The model under review builds one solid part; all positions refer to its coordinate system, in mm. Coordinates: 2 decimals unless noted, no trailing zeros. Write each loop counter-clockwise with the first axis right and the second up, starting at its lowest first coordinate (ties: lowest second). Pieces come first, ordered by that corner, then holes. Notation, with made-up numbers: (63, 11) -> (83, 11) arc R22 cw to (83, 17) -> close; hole circle Ø9 at (84.25, -30.5). An arc over 180 degrees is marked (long way). Put each result on its own line as item: value. Start each with the question number.
from build123d import *


with BuildPart() as part:
    # Sketch1 → Revolve1 (revolve)
    with BuildSketch(Plane(origin=(0, 0, 0), x_dir=(0, 0, -1), z_dir=(1, 0, 0)), mode=Mode.PRIVATE) as revolve1_sk:
        with BuildLine():
            Line((10, 0), (0, 0))
            add(Edge.make_bspline(
                [(0, 0), (3.5599e-05, 0.016666801), (0.000106798, 0.050001231), (0.000652865, 0.100002577), (0.001541965, 0.1500037), (0.00277976, 0.200005118), (0.00437987, 0.250006415), (0.006342127, 0.300007464), (0.008653546, 0.350008586), (0.011306301, 0.400010647), (0.014344795, 0.450011021), (0.017718859, 0.500012898), (0.021465187, 0.550013422), (0.025546859, 0.600015942), (0.030015342, 0.650015894), (0.03482081, 0.70001787), (0.039992041, 0.750019052), (0.045523257, 0.800020171), (0.051408883, 0.850022422), (0.057677216, 0.900021809), (0.064279583, 0.95002496), (0.071264406, 1.000025161), (0.078604568, 1.05002637), (0.086301292, 1.100028717), (0.094377045, 1.150028529), (0.102799423, 1.20003228), (0.111617788, 1.250030975), (0.120783561, 1.300033624), (0.130325404, 1.350034612), (0.140235292, 1.400035949), (0.150516909, 1.450036918), (0.161163804, 1.500039649), (0.17219876, 1.550039155), (0.183594648, 1.600042195), (0.195380444, 1.65004137), (0.207524249, 1.700045854), (0.220069218, 1.750045189), (0.232988482, 1.800046718), (0.246290189, 1.850047612), (0.259968354, 1.900050402), (0.274039825, 1.950051408), (0.288500418, 2.000052634), (0.303351068, 2.050053844), (0.318592454, 2.100054806), (0.334221213, 2.150057651), (0.350251722, 2.200058963), (0.366685967, 2.250057862), (0.383501889, 2.300062903), (0.40073359, 2.350063852), (0.418376737, 2.400063011), (0.436415737, 2.45006601), (0.454864866, 2.500069094), (0.473738026, 2.550068164), (0.493019727, 2.600068939), (0.512706128, 2.650074525), (0.532830884, 2.700072839), (0.553370049, 2.750076061), (0.574338539, 2.800079744), (0.595755257, 2.85007556), (0.61758101, 2.900081863), (0.639854553, 2.950081918), (0.66256348, 3.000085551), (0.685725632, 3.050086231), (0.7093363, 3.100087577), (0.733399151, 3.150087825), (0.757906071, 3.20009433), (0.782892021, 3.250091412), (0.808327595, 3.300098823), (0.834255389, 3.350093071), (0.860630848, 3.400102473), (0.88750378, 3.450102818), (0.914867347, 3.500100816), (0.942705478, 3.550107403), (0.971049019, 3.600107299), (0.999888878, 3.65011121), (1.029241659, 3.70011152), (1.059102526, 3.750114933), (1.089483632, 3.800118313), (1.120396235, 3.850118736), (1.151837467, 3.900122094), (1.183818601, 3.950125628), (1.216352043, 4.000125498), (1.249431788, 4.050132262), (1.283085623, 4.100131924), (1.317306062, 4.150136161), (1.352110512, 4.200135309), (1.387489417, 4.25014553), (1.423484922, 4.300141599), (1.460075424, 4.350148495), (1.497288074, 4.40015156), (1.53513209, 4.450151014), (1.57360284, 4.500160743), (1.612737012, 4.550160216), (1.652530339, 4.600162877), (1.692991663, 4.65017277), (1.734157348, 4.700168226), (1.776008892, 4.750178192), (1.81858317, 4.800180487), (1.861887951, 4.850182262), (1.905930073, 4.900195432), (1.95075691, 4.950189638), (1.996348781, 5.000203486), (2.042755705, 5.050200606), (2.089969588, 5.100213134), (2.13803612, 5.150217143), (2.186971133, 5.200222711), (2.236797623, 5.250226935), (2.287534309, 5.300237945), (2.339222476, 5.350244315), (2.391888284, 5.400253552), (2.445574222, 5.45025529), (2.500276259, 5.500295659), (2.537351737, 5.533372099), (2.55599, 5.55)],
                knots=[0, 0, 0, 0, 0.007942908, 0.015886211, 0.023830326, 0.031775625, 0.039722547, 0.047671504, 0.055622833, 0.063576922, 0.07153435, 0.079495335, 0.087460381, 0.095429767, 0.10340416, 0.111383685, 0.11936889, 0.127360179, 0.135357957, 0.143362824, 0.151374788, 0.159394667, 0.167422653, 0.175459144, 0.183504791, 0.191559748, 0.199624961, 0.207700294, 0.215786437, 0.223883802, 0.231992798, 0.240113836, 0.248247664, 0.256394356, 0.264554679, 0.272728682, 0.280917534, 0.289121281, 0.297340338, 0.305575119, 0.313826467, 0.322094811, 0.330380581, 0.338684203, 0.347006099, 0.355347174, 0.363707867, 0.372088108, 0.380489342, 0.388912021, 0.397356053, 0.405822412, 0.414312099, 0.422825001, 0.431361552, 0.439923369, 0.448510316, 0.457123451, 0.46576386, 0.474430749, 0.483125841, 0.491849606, 0.500603176, 0.50938703, 0.518201646, 0.527047492, 0.535926456, 0.544838318, 0.553785016, 0.56276558, 0.57178273, 0.580836987, 0.589928093, 0.599058103, 0.608227539, 0.617437722, 0.626689183, 0.635983268, 0.645321349, 0.654703976, 0.664132545, 0.673608478, 0.683132339, 0.69270646, 0.702331431, 0.712008739, 0.721738974, 0.731525502, 0.741368016, 0.751269015, 0.761230086, 0.77125187, 0.781337931, 0.791488944, 0.801706572, 0.811994513, 0.822352464, 0.832784196, 0.843291476, 0.853876085, 0.864542998, 0.875291944, 0.886128003, 0.897051998, 0.908069131, 0.919182484, 0.930395179, 0.941710372, 0.953133539, 0.9646691, 0.976321538, 0.988096569, 1, 1, 1, 1], degree=3))
            Line((2.55599, 5.55), (2.55599, 5.75))
            Line((2.55599, 5.75), (3.35748, 5.75))
            Line((3.35748, 5.75), (3.35748, 5.9492))
            ThreePointArc((3.35748, 5.9492), (3.372358976, 5.985121024), (3.40828, 6))
            Line((3.40828, 6), (5.85748, 6))
            Line((5.85748, 6), (5.85748, 5.873))
            Line((5.85748, 5.873), (10.85748, 4.5))
            Line((10.85748, 4.5), (11.35748, 4.5))
            Line((11.35748, 4.5), (11.35748, 3.25))
            add(Edge.make_bspline(
                [(10, 0), (10.000056861, 0.01666708), (10.000170592, 0.0500037), (10.001117916, 0.100007258), (10.002618837, 0.150010821), (10.004729124, 0.20001471), (10.007448952, 0.250018414), (10.010781755, 0.300021674), (10.014713511, 0.350025055), (10.019237073, 0.400029972), (10.024395369, 0.45003214), (10.030142728, 0.500036366), (10.0365002, 0.55004091), (10.043488845, 0.600042391), (10.051062088, 0.650048046), (10.059267779, 0.700050298), (10.068078377, 0.750053759), (10.077497714, 0.800058165), (10.087538544, 0.850061737), (10.098204423, 0.90006334), (10.10946822, 0.950069931), (10.121378341, 1.000069573), (10.1338821, 1.050076401), (10.147029343, 1.100077299), (10.160786514, 1.150082617), (10.175182904, 1.20008343), (10.190190402, 1.250088766), (10.205837242, 1.300089137), (10.222093378, 1.350096132), (10.238998481, 1.400096962), (10.256533003, 1.450097633), (10.27468071, 1.500104385), (10.29347393, 1.550106807), (10.312907874, 1.600107471), (10.332970002, 1.650110027), (10.353661774, 1.700114087), (10.374991067, 1.750119393), (10.396980392, 1.800115743), (10.419583602, 1.85012682), (10.442866046, 1.900119802), (10.46675986, 1.950130895), (10.491328563, 2.000128462), (10.516535034, 2.050137081), (10.542424605, 2.10013211), (10.568950372, 2.150143092), (10.596168084, 2.200140634), (10.624047647, 2.250148072), (10.652620792, 2.300151866), (10.681894818, 2.350153147), (10.711867243, 2.400159359), (10.742558203, 2.450168863), (10.774003866, 2.500169352), (10.806196749, 2.550175824), (10.839159562, 2.600187098), (10.872932785, 2.650196408), (10.907550175, 2.700198383), (10.943011873, 2.750216489), (10.979389434, 2.800226376), (11.016714764, 2.850240931), (11.055043535, 2.900253576), (11.094420826, 2.950276147), (11.134932562, 3.000293776), (11.176645078, 3.05032018), (11.219656781, 3.10034969), (11.264089006, 3.150364301), (11.309969614, 3.200456536), (11.341555497, 3.23339405), (11.35748, 3.25)],
                knots=[0, 0, 0, 0, 0.013871316, 0.027744679, 0.04162207, 0.055505482, 0.069397057, 0.083298853, 0.0972127, 0.11114058, 0.125085031, 0.139047518, 0.15303035, 0.167035925, 0.181065482, 0.195121849, 0.209206593, 0.223321686, 0.237469634, 0.251652447, 0.265871509, 0.28013002, 0.294428661, 0.308770726, 0.323157469, 0.337591571, 0.352074187, 0.366608018, 0.381194123, 0.395836109, 0.410534992, 0.425291675, 0.44010988, 0.454991472, 0.469937257, 0.484948997, 0.500029516, 0.5151817, 0.53040506, 0.545704772, 0.561079045, 0.576533165, 0.59206763, 0.607686658, 0.623389394, 0.639181429, 0.65506315, 0.671038969, 0.687112017, 0.703284041, 0.719559658, 0.735945077, 0.752442192, 0.769055912, 0.785794359, 0.802664341, 0.819669638, 0.836822213, 0.85413113, 0.871607402, 0.88926238, 0.907112993, 0.925174996, 0.943470086, 0.962020759, 0.980852187, 1, 1, 1, 1], degree=3))
        make_face()
    revolve(revolve1_sk.sketch.rotate(Axis((0, 0, -11.886951368), (0, 0, 1)), 90), axis=Axis((0, 0, -11.886951368), (0, 0, 1)))


solid = part.part
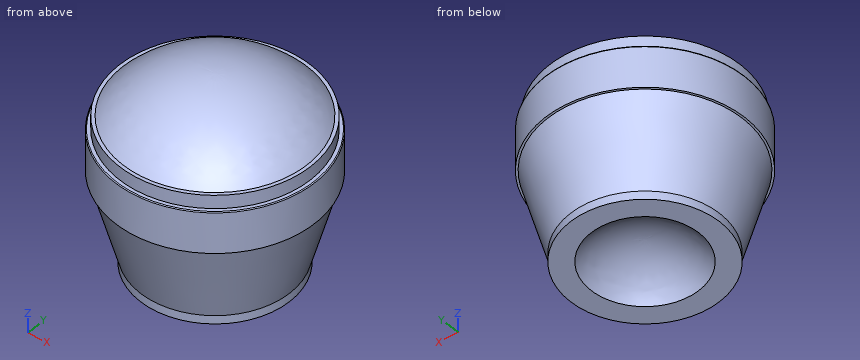
1. Consider section B-B on z = -9. State the section outline as (x, y) points.
2. Wall thickness on line 1 (X direction, y = 0.75, z = -5.5); line 2 (Z direction, x = 3.25, y = 5); line 3 (X direction, y = -3.25, z = -10.5): over which ranges is each line inside the solid? List them lowest first. Write a range as from..to.
3. Insertion check: P1, Ø3.5, axis at x = -1, y = -2.5, coming from the +Z side; P2, Ø1, axis at x = 4.5, z = -2, coming from the +Y side; P3, Ø3, axis at x = 3.5, z = -5, coming from the -Y side. Each pin has a flat end and moves straight along its axis. Give the tip position at first contact, or say it passes through.
4. Consider section A-A on z = -3.75. State the section outline as (x, y) points.
Output values:
1. outline: circle Ø10.02 at (0, 0)
2. line 1: x = -5.95..5.95
2. line 2: z = -5.86..-3.36
2. line 3: x = -3.25..3.25
3. P1: stops at z = -0.06
3. P2: stops at y = 3.41
3. P3: stops at y = -5.66
4. outline: circle Ø12 at (0, 0)
